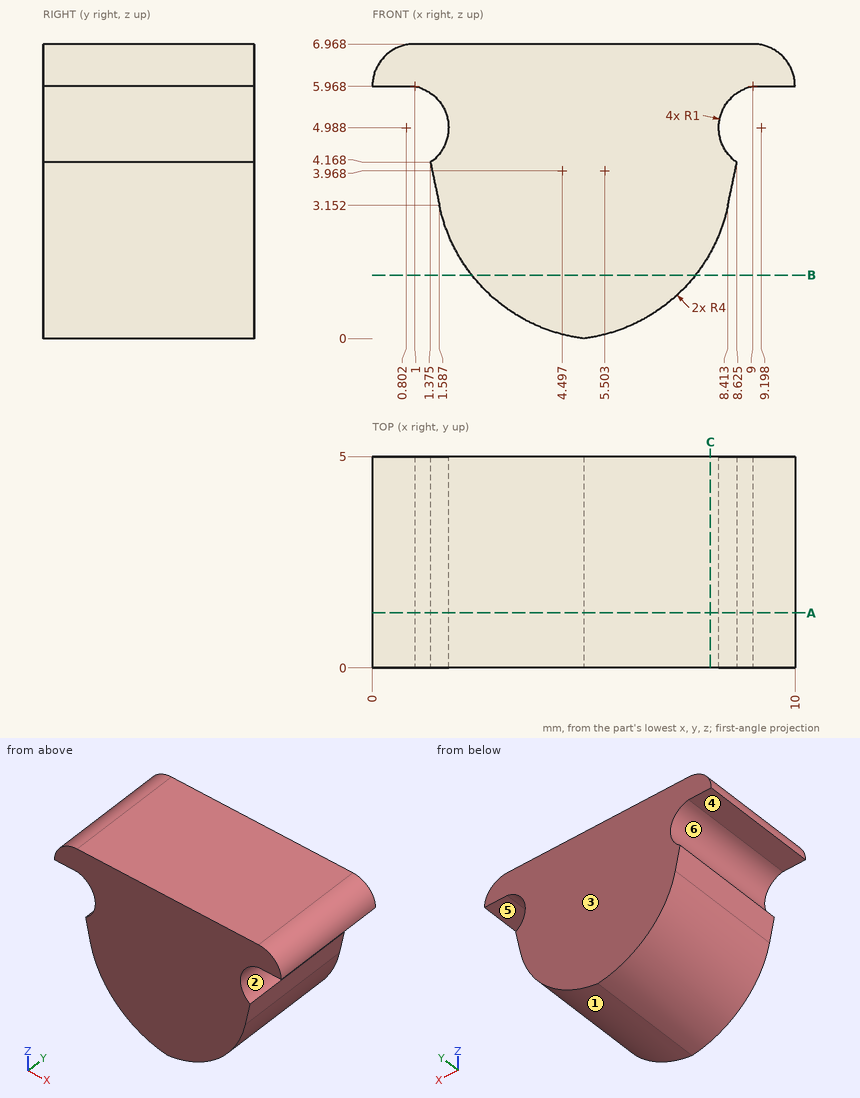
Check sheet for the drawn part. Datum: minimum x, y, z corner. Units: mm. A direction names the side the tool comes from. Coordinates: 2 decimals unless noted, no trailing zeros. Order: outer loops, then holes, each group sorted by start corner. A loop starts at its lowest first (then second) coordinate and runs counter-clockwise, first axis right, second up. Notation, with made-up numbers: (65, -25.5) - (86, -25.5) arc R14 cw to (86, -1.5) - close; hole circle Ø11 at (19.5, 57.5). An arc over 180 degrees is marked (long way). Return JSON: item names as keys, results as strings.
(1) Access from +Z, -Z, +X, -X, +Y, -Y to the whole of each face (thin tool, end or side, straight path). Record for the marked faces 4, 5 and 6.
Filled sheet:
{"face 4": "-Z, -X, +Y, -Y", "face 5": "-Z, +X, +Y, -Y", "face 6": "-X, +Y, -Y"}
(2) Section check C-C, the plane x = 8. Record the cut outline in (y, z).
Filled sheet:
{"outline": "(0, 2.04) - (5, 2.04) - (5, 6.97) - (0, 6.97) - close"}
(3) Section check A-A, the plane y = 1.3. Record the cut outline in (x, z) (1 decimal).
Filled sheet:
{"outline": "(0, 6) - (1, 6) arc R1 cw to (1.4, 4.2) - (1.6, 3.2) arc R4 ccw to (5, 0) arc R4 ccw to (8.4, 3.2) - (8.6, 4.2) arc R1 cw to (9, 6) - (10, 6) arc R1 ccw to (9, 7) - (1, 7) arc R1 ccw to start"}
(4) Section check B-B, the plane z = 1.5. Record the cut outline in (x, y) (1 decimal).
Filled sheet:
{"outline": "(2.4, 0) - (7.6, 0) - (7.6, 5) - (2.4, 5) - close"}
(5) Mould release check, pull along Z, two halves, no side actions. Record for the marked faces 1, 2 and 3: pulls with the +Z half, pulls with the -Z half, needs draft (parallel to the pull), parting line crosses it, or undercut.
Filled sheet:
{"face 1": "pulls with the -Z half", "face 2": "undercut", "face 3": "needs draft"}
(6) Thickness scan on line 1 along X through (y, z) = (1.9, 5); line 2 along Z through (x, y) = (9, 4.2); line 3 along Z through (x, y) = (6.75, 1.4) (1 decimal). Record the ranges inside material, lowest first.
Filled sheet:
{"line 1": "x = 1.8 to 8.2", "line 2": "z = 5.97 to 6.97", "line 3": "z = 0.7 to 7"}
(7) Go/stop test with a flat-tipped pin: pin 1 (0.5 mm diameter, centred on x = 0.5, y = 2.5, fed in from -Z). Record where the tip stops, or that it passes through.
Filled sheet:
{"pin 1": "stops at z = 5.97"}
